Work out the finished part from the listing and answer in its coordinate system (mm). Coordinates: 2 decimals unless noted, no trailing zeros. Write each loop counter-clockwise with the first axis right and the second up, starting at its lowest first coordinate (ties: lowest second). Pieces come first, ordered by that corner, then holes. Notation, with made-up numbers: M -14.75,86 L 16.25,86 A7 ccw 16.25,92 Z; hole C 74,28.25 d1. An arc over 180 degrees is marked long. Use CSV: the item, a comma, the result in double quotes.
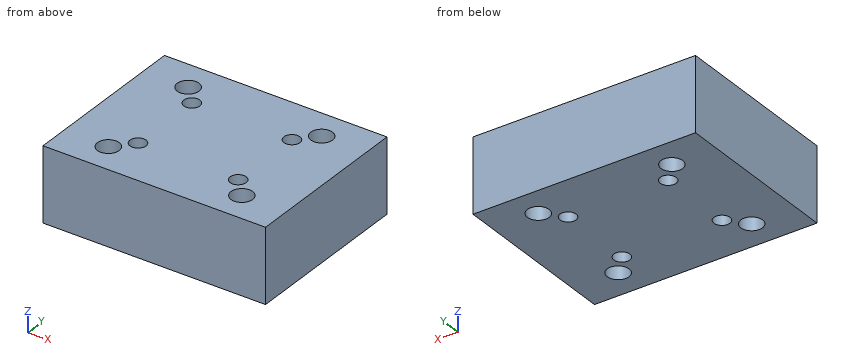
from build123d import *

# Parameters (mm, degrees)
F0_W     = 90
F0_H     = 70
F1_DEPTH = 30
F2_D     = 8.8
F4_D     = 6.5


with BuildPart() as f1:
    # F0 (on Top) → F1 (new body)
    with BuildSketch(Plane.XY):
        with Locations((0, 0.8103642613)):
            Rectangle(F0_W, F0_H)
    extrude(amount=F1_DEPTH)

    # F2 (through all)
    with Locations(Plane(origin=(0, 0, 0), x_dir=(1, 0, 0), z_dir=(0, 0, -1))):
        with Locations((-27, -23.8103642613), (-27, 22.1896357387), (27, 22.1896357387), (27, -23.8103642613)):
            Hole(F2_D / 2)

    # F4 (through all)
    with Locations(Plane.XY.offset(30)):
        with Locations((-20.25, 16.3103642613), (-20.25, -14.6896357387), (20.25, -14.6896357387), (20.25, 16.3103642613)):
            Hole(F4_D / 2)


solid = f1.part
Item 1: Consider probe 1 along Y at (x, z) = (20.25, 22); probe 2 along Y at (x, z) = (-27, 7.5); probe 3 along X at (y, z) = (-22, 10). Determine where each line is inside the solid, lowest interval first.
Answer:
probe 1,"y = -34.19 to -17.94, -11.44 to 13.06, 19.56 to 35.81"
probe 2,"y = -34.19 to -26.59, -17.79 to 19.41, 28.21 to 35.81"
probe 3,"x = -45 to -31.4, -22.6 to 22.6, 31.4 to 45"
Item 2: The part is cut by section A-A (x = 27). Write down the section's boundary in (y, z).
Answer:
outline,"M -34.19,0 L -26.59,0 L -26.59,30 L -34.19,30 Z; M -17.79,0 L 19.41,0 L 19.41,30 L -17.79,30 Z; M 28.21,0 L 35.81,0 L 35.81,30 L 28.21,30 Z"
Item 3: Given pin 1 (10.5 mm diameter, centred on x = -20.25, y = 16.31, fed in from +Z); pin 2 (7 mm diameter, centred on x = 27, y = -22.19, fed in from -Z), each flat-ended and moving along its own axis, determine where each tip first touches the part or whether it passes through.
Answer:
pin 1,"stops at z = 30"
pin 2,"passes through"
Item 4: The part is cut by section C-C (x = -18). Write down the section's boundary in (y, z).
Answer:
outline,"M -34.19,0 L -17.03,0 L -17.03,30 L -34.19,30 Z; M -12.34,0 L 13.97,0 L 13.97,30 L -12.34,30 Z; M 18.66,0 L 35.81,0 L 35.81,30 L 18.66,30 Z"
Item 5: The part is cut by section B-B (z = 3). Count the separate pieces of the cut face and the enclosed holes in it, then the cut area to 3 significant figures.
Answer:
separate pieces,"1"
enclosed holes,"8"
area,"5,920 mm2"
